from build123d import *

# Parameters (mm, degrees)
SKETCH_1_R               = 4.1
EXTRUDE_1_DEPTH          = 10
CUT_EXTRUDE_1_DEPTH      = 10
PATTERN_CIRCULAR_1_COUNT = 3


with BuildPart() as part:
    # 草图1 → 凸台-拉伸1 (new body)
    with BuildSketch(Plane.XY):
        with BuildLine():
            ThreePointArc((-1.339614753, 13.33287037), (-11.604740411, 6.7), (-12.216411823, -5.506294778))
            ThreePointArc((-12.216411823, -5.506294778), (-10.522208656, -6.075), (-10.87679707, -7.826575593))
            ThreePointArc((-10.87679707, -7.826575593), (0, -13.4), (10.87679707, -7.826575593))
            ThreePointArc((10.87679707, -7.826575593), (10.522208656, -6.075), (12.216411823, -5.506294778))
            ThreePointArc((12.216411823, -5.506294778), (11.604740411, 6.7), (1.339614753, 13.33287037))
            ThreePointArc((1.339614753, 13.33287037), (0, 12.15), (-1.339614753, 13.33287037))
        make_face()
        Circle(SKETCH_1_R, mode=Mode.SUBTRACT)
    extrude(amount=EXTRUDE_1_DEPTH)

    # 草图2 → 切除-拉伸1 (cut)
    with BuildSketch(Plane.XY):
        with BuildLine():
            Line((-7.608616423, -6.933177924), (-3.131635256, -4.348391642))
            Line((-3.131635256, -4.348391642), (-1.025, -4.56980793))
            Line((-1.025, -4.56980793), (-1.025, -3.96980793))
            ThreePointArc((-1.025, -3.96980793), (0, -4.1), (1.025, -3.96980793))
            Line((1.025, -3.96980793), (1.025, -4.56980793))
            Line((1.025, -4.56980793), (3.131635256, -4.348391642))
            Line((3.131635256, -4.348391642), (7.608616423, -6.933177924))
            ThreePointArc((7.608616423, -6.933177924), (7.731089256, -7.114227304), (7.664380105, -7.322381963))
            ThreePointArc((7.664380105, -7.322381963), (0, -10.6), (-7.664380105, -7.322381963))
            ThreePointArc((-7.664380105, -7.322381963), (-7.731089256, -7.114227304), (-7.608616423, -6.933177924))
        make_face()
    cut_extrude_1 = extrude(amount=CUT_EXTRUDE_1_DEPTH, mode=Mode.SUBTRACT)

    # 阵列(圆周)1: 切除-拉伸1 ×3 about axis
    pattern_circular_1_axis = Axis((0, 0, 0), (0, 0, 1))
    for i in range(1, PATTERN_CIRCULAR_1_COUNT):
        add(cut_extrude_1.rotate(pattern_circular_1_axis, i * 360 / PATTERN_CIRCULAR_1_COUNT), mode=Mode.SUBTRACT)


solid = part.part
The listing builds one solid part. Answer for the finished solid, in the listing's coordinates (mm). A direction names the side the tool comes from. Give positions to 0.01 mm unless a question says otherwise; leave off trailing zeros. Write each loop counter-clockwise with the first axis right and the second up, starting at its lowest first coordinate (ties: lowest second). Pieces come first, ordered by that corner, then holes. Notation, with made-up numbers: (66, -8) -> (108, -8) arc R7 cw to (108, 1) -> close; hole circle Ø1 at (72, -31.75). An arc over 180 degrees is marked (long way). One line per question, with ' | ' between items. Start each with the question number.
1. For a pull along Y with two mould halves and no side action, classify faces 1 (the flat face through (-3.2, -2.8, 0)), 2 (the cylindrical face through (-0.2, -13.4, 4.9)), 3 (the cylindrical face through (0, 4.1, 4.9)) as pulls with the +Y half, pulls with the -Y half, needs draft (parallel to the pull), parting line crosses it, or undercut.
2. Given pin 1 Ø5.5 at (y, z) = (7, 5) entering from -X; pin 2 Ø6 at (x, z) = (-3.5, 4.5) entering from -Y; pin 3 Ø5.5 at (y, z) = (8.5, 7) entering from +X, each flat-ended and moving along its own axis, determine where each tip first touches the part or whether it passes through.
3. For faces 4 (the cylindrical face through (11.69, 6.55, 4.93)), 5 (the flat face through (-4.895, 0.443, 4.93)), determine the directions among +Z, -Z, +X, -X, +Y, -Y from which every point of the face is accessible in a straight line to the end or side of a thin tool.
4. Section C-C (y = -8.5) is taken. Determine the outline of the cut face in (x, z), plus the area to 3 significant figures.
5. Find the intervals of material crossed by probe 1 along Y at (x, z) = (-6.75, 0.75); probe 2 along X at (y, z) = (8.25, 1); probe 3 along Y at (x, z) = (-7.5, 6.75), in increasing order.
6. Section B-B (x = 9.25) is taken. Determine the outline of the cut face in (y, z).
7. Section D-D (x = -6.25) is taken. Determine the outline of the cut face in (y, z), plus the area to 3 significant figures.
8. Section A-A (y = 3.5) is taken. Determine the outline of the cut face in (x, z), plus the area to 3 significant figures.
Response values:
1) face 1: needs draft | face 2: pulls with the -Y half | face 3: undercut
2) pin 1: x = -12.71 | pin 2: y = -13.39 | pin 3: x = 12.1
3) face 4: +Z, -Z, +X | face 5: +Z, -Z
4) outline: (-10.36, 0) -> (-6.33, 0) -> (-6.33, 10) -> (-10.36, 10) -> close; (6.33, 0) -> (10.36, 0) -> (10.36, 10) -> (6.33, 10) -> close | area: 80.5 mm2
5) probe 1: -11.58 to -8.17, -6.44 to -1.36, 8.17 to 11.58 | probe 2: -10.56 to -6.66, -2.2 to 2.2, 6.66 to 10.56 | probe 3: -11.1 to -7.49, -6.87 to -1.79, 7.49 to 11.1
6) outline: (-9.7, 0) -> (-2.8, 0) -> (-2.8, 10) -> (-9.7, 10) -> close; (5.18, 0) -> (9.7, 0) -> (9.7, 10) -> (5.18, 10) -> close
7) outline: (-11.85, 0) -> (-8.56, 0) -> (-8.56, 10) -> (-11.85, 10) -> close; (-6.15, 0) -> (-1.07, 0) -> (-1.07, 10) -> (-6.15, 10) -> close; (8.56, 0) -> (11.85, 0) -> (11.85, 10) -> (8.56, 10) -> close | area: 117 mm2
8) outline: (-12.93, 0) -> (-10.01, 0) -> (-10.01, 10) -> (-12.93, 10) -> close; (-3.21, 0) -> (-2.14, 0) -> (-2.14, 10) -> (-3.21, 10) -> close; (2.14, 0) -> (3.21, 0) -> (3.21, 10) -> (2.14, 10) -> close; (10.01, 0) -> (12.93, 0) -> (12.93, 10) -> (10.01, 10) -> close | area: 80.0 mm2
